```python
from build123d import *

# Parameters (mm, degrees)
SALIENTE_EXTRUIR1_DEPTH = 3


with BuildPart() as part:
    # Model → Saliente-Extruir1 (new body)
    with BuildSketch(Plane.XY):
        with BuildLine():
            Line((52.126339564, 0.69142602), (71.859672897, 0.69142602))
            Line((71.859672897, 0.69142602), (71.859672897, 5.69142602))
            ThreePointArc((71.859672897, 5.69142602), (73.216437638, 11.459046612), (76.864886687, 16.127566441))
            ThreePointArc((76.864886687, 16.127566441), (78.358673415, 24.066839848), (70.578789676, 26.243275014))
            ThreePointArc((70.578789676, 26.243275014), (67.341569383, 25.013085855), (63.940045397, 24.363012656))
            Line((63.940045397, 24.363012656), (63.937229303, 26.362731754))
            Line((63.937229303, 26.362731754), (66.030265375, 28.484052098))
            Line((66.030265375, 28.484052098), (62.541871922, 32.019586004))
            ThreePointArc((62.541871922, 32.019586004), (61.844193231, 32.30857398), (61.14651454, 32.019586004))
            Line((61.14651454, 32.019586004), (57.658121086, 28.484052098))
            Line((57.658121086, 28.484052098), (59.990562636, 26.362731754))
            Line((59.990562636, 26.362731754), (59.990562636, 24.368482398))
            ThreePointArc((59.990562636, 24.368482398), (56.626825565, 25.017616984), (53.424360475, 26.234301063))
            ThreePointArc((53.424360475, 26.234301063), (45.632437064, 24.074933253), (47.121132781, 16.127561055))
            ThreePointArc((47.121132781, 16.127561055), (48.940005662, 14.312179557), (50.391114233, 12.191285299))
            ThreePointArc((50.391114233, 12.191285299), (51.660499902, 9.048614396), (52.126339564, 5.69142602))
            Line((52.126339564, 5.69142602), (52.126339564, 0.69142602))
        make_face()
        with BuildLine():
            Line((59.990562636, 22.359186797), (59.990562636, 5.69142602))
            Line((59.990562636, 5.69142602), (54.098159046, 5.69142602))
            ThreePointArc((54.098159046, 5.69142602), (52.556239166, 12.312269616), (48.376647716, 17.673622257))
            ThreePointArc((48.376647716, 17.673622257), (47.306956592, 22.997651717), (52.54077152, 24.445653821))
            ThreePointArc((52.54077152, 24.445653821), (56.172655621, 23.070320202), (59.990562636, 22.359186797))
        make_face(mode=Mode.SUBTRACT)
        with BuildLine():
            Line((63.966339564, 5.69142602), (63.942873914, 22.354472252))
            ThreePointArc((63.942873914, 22.354472252), (67.795799116, 23.065868121), (71.459909133, 24.453461173))
            ThreePointArc((71.459909133, 24.453461173), (76.670564355, 23.010720068), (75.647074312, 17.701774987))
            ThreePointArc((75.647074312, 17.701774987), (71.439696493, 12.333149563), (69.886739491, 5.69142602))
            Line((69.886739491, 5.69142602), (63.966339564, 5.69142602))
        make_face(mode=Mode.SUBTRACT)
    extrude(amount=SALIENTE_EXTRUIR1_DEPTH)


solid = part.part
```
CAD build for the part. Positions are in the model's coordinates, mm. A direction names the side the tool comes from. Give positions to 0.01 mm unless a question says otherwise; leave off trailing zeros. Order: outer loops, then holes, each group sorted by start corner. A loop starts at its lowest first (then second) coordinate and runs counter-clockwise, first axis right, second up. Notation, with made-up numbers: M -34.75,63 L 10.25,63 A17 ccw 10.25,90 Z; hole C 52,-5.75 d3. An arc over 180 degrees is marked long. Put each result on its own line as item: value. Start each with the question number.
(1) Saw through at C-C, the plane z = 2.15. Write the cut outline in (x, y).
(2) Which spindle directions (+Z, -Z, +X, -X, +Y, -Y) get a long thin tool onto all of the face, cutting with end or side? Do faces 1 (the flat face through (59.43, 30.28, 1.48)), 2 (the cylindrical face through (67.74, 23.05, 1.48)). Say none if no direction does.
(3) Saw through at A-A, the plane y = 19.5. Write the cut outline in (x, z), then the cut area to 3 significant figures.
(4) Saw through at B-B, the plane x = 48. Write the cut outline in (y, z), then the cut area to 3 significant figures.
(5) Saw through at D-D, the plane y = 23. Write the cut outline in (x, z).
(6) Mould opens along Y. For faces 3 (the flat face through (52.126, 3, 1)), 4 (the flat face through (67, 5.691, 1)), 5 (the flat face through (64.31, 30.23, 1.48)) say: +Y half, -Y half, draft (parallel to the pull), parting line (faces both ways), or undercut.
(7) Flat gauge pins, fed straight in: pin 1 Ø0.9 at (x, z) = (58, 2) entering from +Y; pin 2 Ø1.5 at (y, z) = (26, 0.5) entering from -X; pin 3 Ø0.9 at (y, z) = (3, 2) entering from -X; pin 4 Ø1.5 at (x, y) = (53, 29) entering from -Z. Where does each tip first touch, or does it go through?
(8) Drill centre lines: line 1 along X through (y, z) = (6, 2.15); line 2 along X through (y, z) = (14, 1.65); line 3 along Y through (x, z) = (58, 1.55). Where is each one in solid material? Low to high.
Check result:
1. outline: M 47.12,16.13 A13.81 cw 52.13,5.69 L 52.13,0.69 L 71.86,0.69 L 71.86,5.69 A13.81 cw 76.86,16.13 A5.98 ccw 70.58,26.24 A19.89 cw 63.94,24.36 L 63.94,26.36 L 66.03,28.48 L 62.54,32.02 A0.99 ccw 61.15,32.02 L 57.66,28.48 L 59.99,26.36 L 59.99,24.37 A19.89 cw 53.42,26.23 A5.98 ccw Z; hole M 48.38,17.67 A15.81 cw 54.1,5.69 L 59.99,5.69 L 59.99,22.36 A21.87 cw 52.54,24.45 A3.99 ccw Z; hole M 63.94,22.35 L 63.97,5.69 L 69.89,5.69 A15.8 cw 75.65,17.7 A3.98 ccw 71.46,24.45 A21.87 cw Z
2. face 1: +Z, -Z, -X, +Y
2. face 2: +Z, -Z
3. outline: M 44.9,0 L 46.97,0 L 46.97,3 L 44.9,3 Z; M 59.99,0 L 63.95,0 L 63.95,3 L 59.99,3 Z; M 77.01,0 L 79.09,0 L 79.09,3 L 77.01,3 Z
3. area: 24.3 mm2
4. outline: M 15.33,0 L 17.98,0 L 17.98,3 L 15.33,3 Z; M 23.84,0 L 26.24,0 L 26.24,3 L 23.84,3 Z
4. area: 15.1 mm2
5. outline: M 45.1,0 L 47.31,0 L 47.31,3 L 45.1,3 Z; M 56.43,0 L 67.55,0 L 67.55,3 L 56.43,3 Z; M 76.68,0 L 78.88,0 L 78.88,3 L 76.68,3 Z
6. face 3: draft
6. face 4: undercut
6. face 5: +Y half
7. pin 1: stops at y = 29.29
7. pin 2: stops at x = 46.59
7. pin 3: stops at x = 52.13
7. pin 4: passes through
8. line 1: x = 52.12 to 54.09, 59.99 to 63.97, 69.89 to 71.87
8. line 2: x = 49.19 to 51.62, 59.99 to 63.95, 72.37 to 74.79
8. line 3: y = 0.69 to 5.69, 22.64 to 24.68, 28.17 to 28.83
